Design review of the part built by this model. Coordinates are the model's own, in mm. Face numbers are marked on the shaded views. A direction names the side the tool comes from. Coordinates: 2 decimals unless noted, no trailing zeros. Write each loop counter-clockwise with the first axis right and the second up, starting at its lowest first coordinate (ties: lowest second). Pieces come first, ordered by that corner, then holes. Notation, with made-up numbers: (51, -2.75) - (85, -2.75) arc R23 ccw to (85, 31.25) - close; hole circle Ø5 at (-9.75, 28). An arc over 180 degrees is marked (long way). Answer as a JSON object with one key per item and string values.
```python
from build123d import *

# Parameters (mm, degrees)
BOSS_EXTRUDE1_DEPTH = 7.62
CUT_EXTRUDE1_DEPTH  = 7.62


with BuildPart() as part:
    # Sketch1 → Boss-Extrude1 (new, symmetric)
    with BuildSketch(Plane.XY):
        with BuildLine():
            ThreePointArc((31.75, 0), (0, 31.75), (-31.75, 0))
            Line((-31.75, 0), (31.75, 0))
        make_face()
    extrude(amount=BOSS_EXTRUDE1_DEPTH, both=True)

    # Sketch2 → Cut-Extrude1 (cut)
    with BuildSketch(Plane.XY):
        with BuildLine():
            ThreePointArc((17.78, 26.304640275), (0, 31.75), (-17.78, 26.304640275))
            Line((-17.78, 26.304640275), (-17.78, 7.62))
            Line((-17.78, 7.62), (17.78, 7.62))
            Line((17.78, 7.62), (17.78, 26.304640275))
        make_face()
    extrude(amount=-CUT_EXTRUDE1_DEPTH, mode=Mode.SUBTRACT)


solid = part.part
```
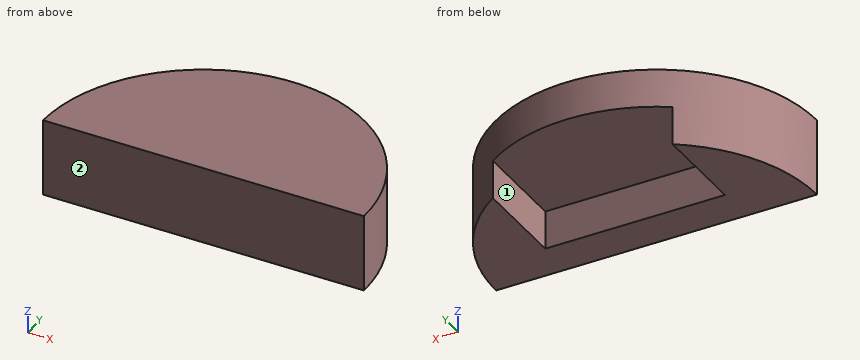
(1) To check wall thickness, follow line 1 (Y direction, x = -7.5, z = -5); line 2 (X direction, y = 12.5, z = -3.5); line 3 (X direction, y = 22, z = -5.25). State the ranges of each line that lie inside material, in increasing order. Write a range as from..to.
Solved:
{"line 1": "y = 0..7.62", "line 2": "x = -29.19..-17.78, 17.78..29.19", "line 3": "x = -22.89..-17.78, 17.78..22.89"}
(2) Take a section at B-B, the plane x = 0. Write out the cut boundary in (y, z).
Solved:
{"outline": "(0, -7.62) - (7.62, -7.62) - (7.62, 0) - (31.75, 0) - (31.75, 7.62) - (0, 7.62) - close"}
(3) Take a section at D-D, the plane z = 2.5. Write out the cut boundary in (x, y).
Solved:
{"outline": "(-31.75, 0) - (31.75, 0) arc R31.75 ccw to start"}
(4) For pin 1 (6 mm diameter, centred on y = 16.5, z = -3.5, fed in from -X); pin 2 (5 mm diameter, centred on y = 24, z = 5.5, fed in from -X); pin 3 (3 mm diameter, centred on y = 15, z = 1, fed in from +X), all flat-tipped, find the tip position at first contact; note any pin that passes through.
Solved:
{"pin 1": "stops at x = -28.74", "pin 2": "stops at x = -23.36", "pin 3": "stops at x = 28.74"}
(5) Take a section at C-C, the plane z = -2. Write out the cut boundary in (x, y), and give its area (3 significant figures).
Solved:
{"outline": "(-31.75, 0) - (31.75, 0) arc R31.75 ccw to (17.78, 26.3) - (17.78, 7.62) - (-17.78, 7.62) - (-17.78, 26.3) arc R31.75 ccw to start", "area": "788 mm^2"}
(6) Tool access review of the marked faces 1 and 2: name each direction out of +Z, -Z, +X, -X, +Y, -Y from which nothing blocks a thin tool from reaching the whole face with its end or side.
Solved:
{"face 1": "-Z, +Y", "face 2": "+Z, -Z, +X, -X, -Y"}
(7) Take a section at A-A, the plane y = 21.5. Write out the cut boundary in (x, z).
Solved:
{"outline": "(-23.36, -7.62) - (-17.78, -7.62) - (-17.78, 0) - (17.78, 0) - (17.78, -7.62) - (23.36, -7.62) - (23.36, 7.62) - (-23.36, 7.62) - close"}
